```python
from build123d import *

# Parameters (mm, degrees)
ENL_V_MAT_EXTRU_1_DEPTH      = 172.053325019
ENL_V_MAT_EXTRU_1_DEPTH_BACK = 172.053325019
ESQUISSE2_W                  = 30
ESQUISSE2_H                  = 12
ENL_V_MAT_EXTRU_2_DEPTH      = 172.928008189
ENL_V_MAT_EXTRU_2_DEPTH_BACK = 172.928008189
ESQUISSE3_R                  = 3


with BuildPart() as part:
    # Esquisse1 → Révolution1 (revolve)
    with BuildSketch(Plane.XY, mode=Mode.PRIVATE) as r_volution1_sk:
        Polygon((40, 3), (0, 3), (0, 15.85), (25.2, 15.85), (25.2, 22), (52.2, 22), (52.2, 20), (128.2, 20), (128.2, 22), (168.2, 22), (168.2, 0), (40, 0), align=None)
    revolve(r_volution1_sk.sketch.rotate(Axis((40, 0, 0), (1, 0, 0)), 180), axis=Axis((40, 0, 0), (1, 0, 0)))

    # Esquisse2 → Enlèv. mat.-Extru.1 (cut, two sides: drawn at the far end of the back side and taken through both)
    with BuildSketch(Plane(origin=(0, 0, 0), x_dir=(1, 0, 0), z_dir=(0, 1, 0)).offset(-ENL_V_MAT_EXTRU_1_DEPTH_BACK)):
        with Locations((153.2, 0)):
            Rectangle(ESQUISSE2_W, ESQUISSE2_H)
    extrude(amount=ENL_V_MAT_EXTRU_1_DEPTH + ENL_V_MAT_EXTRU_1_DEPTH_BACK, mode=Mode.SUBTRACT)

    # Esquisse3 → Enlèv. mat.-Extru.2 (cut, two sides: drawn at the far end of the back side and taken through both)
    with BuildSketch(Plane.XY.offset(-6).offset(-ENL_V_MAT_EXTRU_2_DEPTH_BACK)):
        with Locations((153.2, 0)):
            Circle(ESQUISSE3_R)
    extrude(amount=ENL_V_MAT_EXTRU_2_DEPTH + ENL_V_MAT_EXTRU_2_DEPTH_BACK, mode=Mode.SUBTRACT)


solid = part.part
```
For this review, take the finished solid that the model builds, in its own axes (mm). A direction names the side the tool comes from. Round coordinates to 2 decimals unless told otherwise and drop trailing zeros. Write each loop counter-clockwise with the first axis right and the second up, starting at its lowest first coordinate (ties: lowest second). Pieces come first, ordered by that corner, then holes. Notation, with made-up numbers: (80, -3.75) - (96, -3.75) arc R27 cw to (96, 35.25) - close; hole circle Ø7 at (41.5, -30.75). An arc over 180 degrees is marked (long way). Answer as a JSON object with one key per item and string values.
1. To check wall thickness, follow line 1 along X through (y, z) = (0, 17.75); line 2 along Z through (x, y) = (25.5, 0); line 3 along X through (y, z) = (0, -10). State the ranges of each line that lie inside material, in increasing order.
Response values:
{"line 1": "x = 25.2 to 150.2, 156.2 to 168.2", "line 2": "z = -22 to -3, 3 to 22", "line 3": "x = 0 to 150.2, 156.2 to 168.2"}
2. For pin 1 Ø3.5 at (y, z) = (-5.5, 0) entering from +X; pin 2 Ø1.5 at (x, z) = (45.5, -7.5) entering from +Y; pin 3 Ø3 at (x, z) = (59, -1) entering from +Y, all flat-tipped, find the tip position at first contact; note any pin that passes through.
Response values:
{"pin 1": "stops at x = 138.2", "pin 2": "stops at y = 20.94", "pin 3": "stops at y = 20"}
3. We need section A-A on y = 0. Count the separate pieces of the cut face and the enclosed holes in it, then the cut area to 3 significant figures.
Response values:
{"separate pieces": "3", "enclosed holes": "0", "area": "5,990 mm2"}
4. Draft analysis for pull direction Z (two halves, no side actions). For faces 1 (the face through (150, 0, -6)), 2 (the face through (19.72, -2.86, -0.9)), 3 (the face through (156.06, 0.9, -14.11)), 4 (the face through (148.48, -20.32, 8.43)), state which applies: +Z half, -Z half, draft (parallel to the pull), parting line (faces both ways), or undercut.
Response values:
{"face 1": "undercut", "face 2": "undercut", "face 3": "draft", "face 4": "parting line"}
5. We need section C-C on z = -11. Give the boundary of the cut face in (x, y), then the cut area to 3 significant figures.
Response values:
{"outline": "(0, -11.41) - (25.2, -11.41) - (25.2, -19.05) - (52.2, -19.05) - (52.2, -16.7) - (128.2, -16.7) - (128.2, -19.05) - (168.2, -19.05) - (168.2, 19.05) - (128.2, 19.05) - (128.2, 16.7) - (52.2, 16.7) - (52.2, 19.05) - (25.2, 19.05) - (25.2, 11.41) - (0, 11.41) - close; hole circle Ø6 at (153.2, 0)", "area": "5,640 mm2"}
6. We need section D-D on x = 158. Give the boundary of the cut face in (y, z).
Response values:
{"outline": "(-21.17, -6) arc R22 ccw to (21.17, -6) - close; (-21.17, 6) - (21.17, 6) arc R22 ccw to start"}
7. We need section B-B on z = 0. Give the boundary of the cut face in (x, y).
Response values:
{"outline": "(0, -15.85) - (25.2, -15.85) - (25.2, -22) - (52.2, -22) - (52.2, -20) - (128.2, -20) - (128.2, -22) - (138.2, -22) - (138.2, 22) - (128.2, 22) - (128.2, 20) - (52.2, 20) - (52.2, 22) - (25.2, 22) - (25.2, 15.85) - (0, 15.85) - (0, 3) - (40, 3) - (40, -3) - (0, -3) - close"}
8. Tool access review of faces 5 (the face through (52.2, -10, 18)), 6 (the face through (168.2, 0, 12)), 7 (the face through (25.2, 14, 9)), 8 (the face through (0, 3.3, -0.2)), 9 (the face through (150, 0, 6)): name each direction out of +Z, -Z, +X, -X, +Y, -Y from which nothing blocks a thin tool from reaching the whole face with its end or side.
Response values:
{"face 5": "none", "face 6": "+Z, -Z, +X, +Y, -Y", "face 7": "-X", "face 8": "+Z, -Z, -X, +Y, -Y", "face 9": "+X, +Y, -Y"}
